Could you check a few things on this model? Use its own coordinates, in mm. A direction names the side the tool comes from. Give positions to 0.01 mm unless a question says otherwise; leave off trailing zeros. Order: outer loops, then holes, each group sorted by start corner. A loop starts at its lowest first (then second) coordinate and runs counter-clockwise, first axis right, second up. Notation, with made-up numbers: (-39, 67) - (-6, 67) arc R21 ccw to (-6, 74) - close; hole circle Ø8 at (21, 20). An arc over 180 degrees is marked (long way). One line per question, with ' | ' between items. Start each with the question number.
1. Imagine slicing it at B-B (z = 4.05). Please give me the cut outline in (x, y).
2. Imagine slicing it at D-D (y = -15). Please give me the cut outline in (x, z).
3. Imagine slicing it at C-C (x = -10.5). Please give me the cut outline in (y, z).
4. If we mould it in two halves opening along X, with no side actions, what happens to faces 3 (the flat face through (-12.451, 23, 3)), 4 (the flat face through (-22, 25.311, 3)), 5 (the cylindrical face through (-28.722, -16.213, 2.704))? For each: released by +X, released by -X, zero draft, split by the parting line, or undercut.
5. Which directions (+Z, -Z, +X, -X, +Y, -Y) give clear straight access to the entire face, cutting with the end or side of a thin tool? Please do faces 1 (the flat face through (-4, 4, 5.334)), 2 (the flat face through (5.686, 23, 3)).
6. Imagine slicing it at A-A (y = 21.5). Please give me the cut outline in (x, z).
7. I need wall thicknesses on probe 1 along X at (y, z) = (21, 0.2); probe 2 along Y at (x, z) = (-9, 1.55); probe 3 along Y at (x, z) = (21, 3.85). Which ranges of each line are inside material? Lowest first, please. Write a range as from..to.
```python
from build123d import *

# Parameters (mm, degrees)
SKETCH1_W           = 54.356
SKETCH1_H           = 43.434
BOSS_EXTRUDE1_DEPTH = 5.334
SKETCH2_W           = 18.137033298
SKETCH2_H           = 5.334
CUT_EXTRUDE1_DEPTH  = 41.016719041
FILLET1_R           = 6.35


with BuildPart() as part:
    # Sketch1 → Boss-Extrude1 (new body)
    with BuildSketch(Plane.XY):
        with Locations((-3.35450847, 3.594107707)):
            Rectangle(SKETCH1_W, SKETCH1_H)
    extrude(amount=BOSS_EXTRUDE1_DEPTH)

    # Sketch2 → Cut-Extrude1 (cut, through all)
    with BuildSketch(Plane.XY.offset(5.334)):
        with Locations((-3.382058417, 22.644107707)):
            Rectangle(SKETCH2_W, SKETCH2_H)
    extrude(amount=-CUT_EXTRUDE1_DEPTH, mode=Mode.SUBTRACT)

    # Fillet1
    fillet1_edges = [part.edges().sort_by_distance(p)[0] for p in [
        (23.82349153, -18.122892293, 2.667),
        (-30.53250847, -18.122892293, 2.667),
    ]]
    fillet(fillet1_edges, radius=FILLET1_R)


solid = part.part
```
Results found:
1) outline: (-30.53, -11.77) arc R6.35 ccw to (-24.18, -18.12) - (17.47, -18.12) arc R6.35 ccw to (23.82, -11.77) - (23.82, 25.31) - (5.69, 25.31) - (5.69, 19.98) - (-12.45, 19.98) - (-12.45, 25.31) - (-30.53, 25.31) - close
2) outline: (-29.65, 0) - (22.94, 0) - (22.94, 5.33) - (-29.65, 5.33) - close
3) outline: (-18.12, 0) - (19.98, 0) - (19.98, 5.33) - (-18.12, 5.33) - close
4) face 3: undercut | face 4: zero draft | face 5: released by -X
5) face 1: +Z, +X, -X, +Y, -Y | face 2: +Z, -Z, +Y
6) outline: (-30.53, 0) - (-12.45, 0) - (-12.45, 5.33) - (-30.53, 5.33) - close; (5.69, 0) - (23.82, 0) - (23.82, 5.33) - (5.69, 5.33) - close
7) probe 1: x = -30.53..-12.45, 5.69..23.82 | probe 2: y = -18.12..19.98 | probe 3: y = -17.05..25.31
